Input: dimensioned drawing with shaded views. Units: mm. Origin: part minimum x, y, z. A direction names the side the tool comes from. Coordinates: 2 decimals unless noted, no trailing zeros. Loops run counter-clockwise (first coordinate to the right, second up) from the corner with the lowest first, then second, coordinate; pieces in that order, holes last.
Item 1: Section query B-B, the plane z = 0.55. State how many separate pieces and enclosed holes the cut face has, then the cut area to 3 significant figures.
Item 2: Line query: probe 1 along Y at (x, z) = (10.5, 1.8); probe 2 along Y at (x, z) = (12, 1.5) (1 decimal); probe 3 along X at (y, z) = (10, 2.2). Output: solid intervals per line, ascending.
Item 3: Section query C-C, the plane x = 10.5. Return the cut outline in (y, z), then the cut area to 3 significant figures.
Item 4: Pull-direction query (Y, two-part tool) for the marked faces 1, 2 and 3; classes: +Y half, -Y half, draft (parallel to the pull), parting line (faces both ways), or undercut.
Item 5: Section query D-D, the plane x = 2. Return the cut outline in (y, z).
Item 6: Pin query (flat end, axial travel): pin 1 Ø1 at (y, z) = (25, 2.5) entering from +X; pin 2 Ø0.9 at (x, z) = (2, 1) entering from -Y; pin 3 Ø1.5 at (y, z) = (12.5, 1) entering from -X. Return the tip coordinate at first contact, or that it passes through.
Item 7: Reachability of the marked faces 4, 5 and 6 from +Z, -Z, +X, -X, +Y, -Y: full face, straight path, thin tool, end or side. Return the list, or none.
Item 8: Section query A-A, the plane y = 4.7. Return the cut outline in (x, z), then the cut area to 3 significant figures.
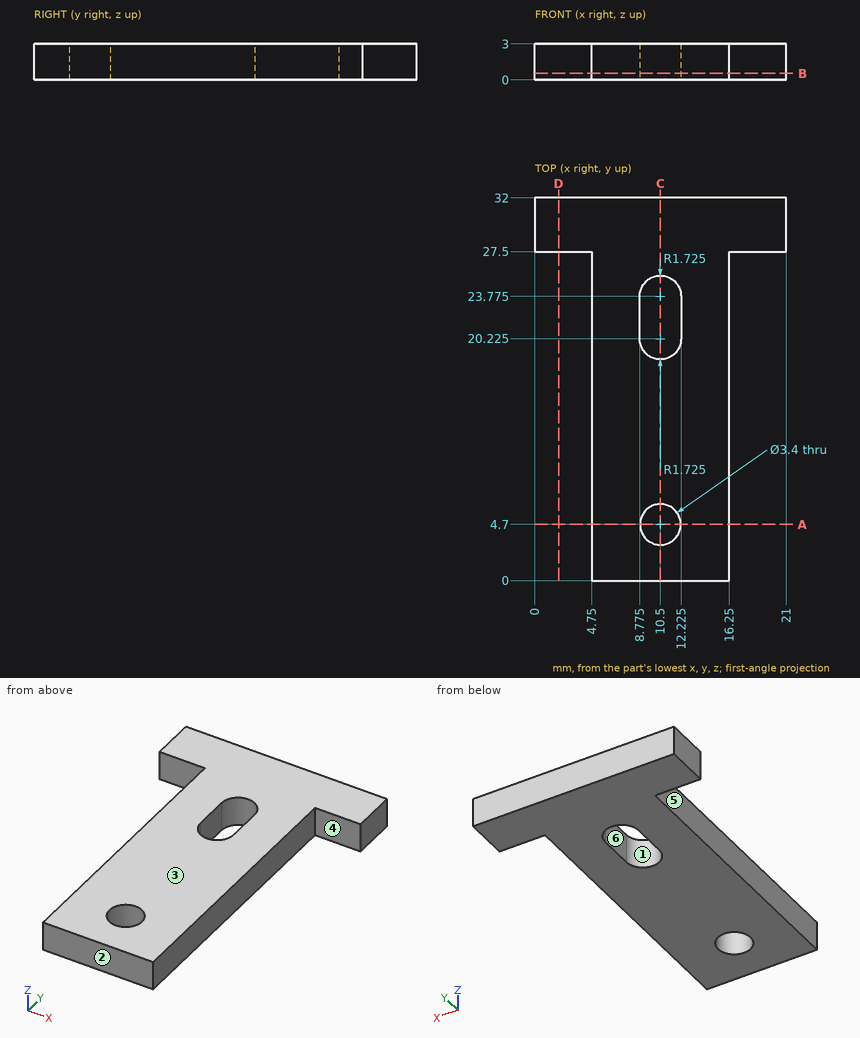
Verdict:
1. separate pieces: 1
1. enclosed holes: 2
1. area: 380 mm2
2. probe 1: y = 0 to 3, 6.4 to 18.5, 25.5 to 32
2. probe 2: y = 0 to 3.9, 5.5 to 19.4, 24.6 to 32
2. probe 3: x = 4.75 to 16.25
3. outline: (0, 0) - (3, 0) - (3, 3) - (0, 3) - close; (6.4, 0) - (18.5, 0) - (18.5, 3) - (6.4, 3) - close; (25.5, 0) - (32, 0) - (32, 3) - (25.5, 3) - close
3. area: 64.8 mm2
4. face 1: undercut
4. face 2: -Y half
4. face 3: draft
5. outline: (27.5, 0) - (32, 0) - (32, 3) - (27.5, 3) - close
6. pin 1: stops at x = 16.25
6. pin 2: stops at y = 27.5
6. pin 3: stops at x = 4.75
7. face 4: +Z, -Z, +X, -Y
7. face 5: +Z, -Z, -X, -Y
7. face 6: +Z, -Z
8. outline: (4.75, 0) - (8.8, 0) - (8.8, 3) - (4.75, 3) - close; (12.2, 0) - (16.25, 0) - (16.25, 3) - (12.2, 3) - close
8. area: 24.3 mm2
